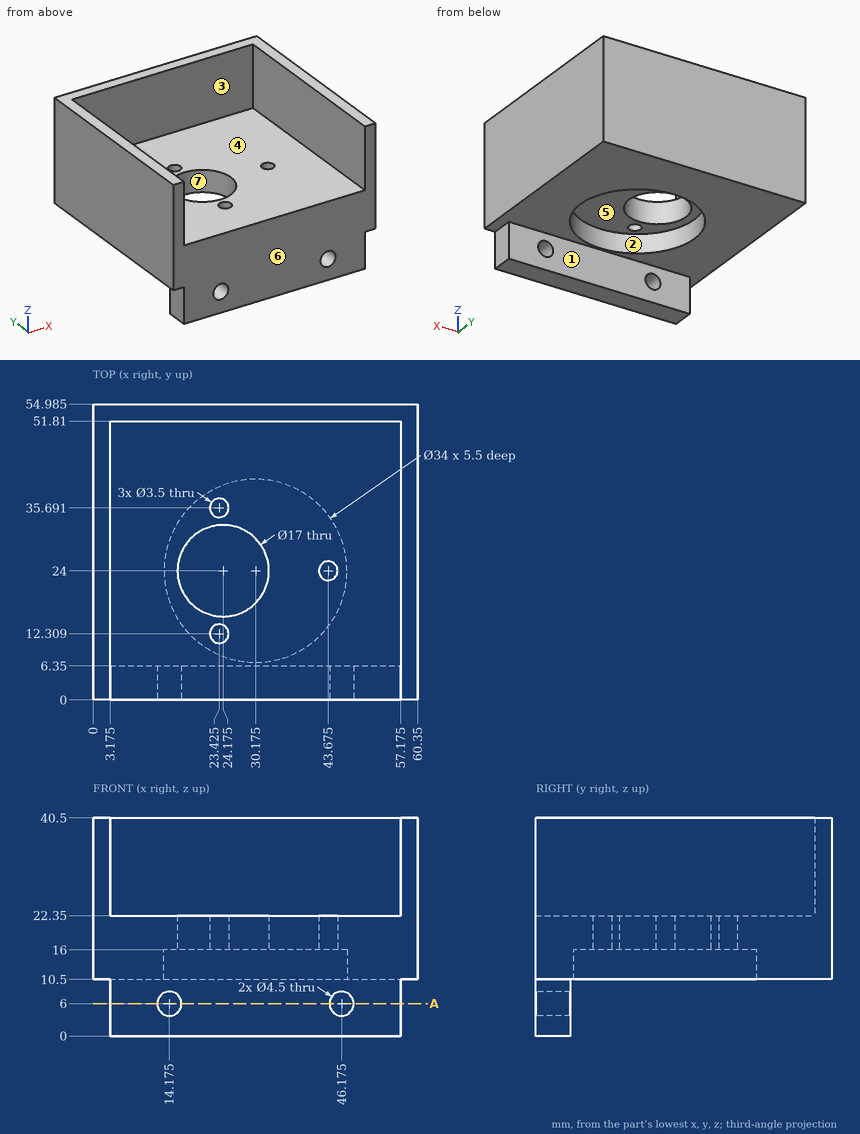
Geometry check sheet. Reference: drawing and pictorial views, mm from the part's lowest x, y, z. A direction names the side the tool comes from. Coordinates: 2 decimals unless noted, no trailing zeros. Write item = value, one per line. Start each with the question number.
1. Mould release check, pull along Y, two halves, no side actions. Record for the marked faces 4, 5, 6 and 7: pulls with the +Y half, pulls with the -Y half, needs draft (parallel to the pull), parting line crosses it, or undercut.
2. Sectioned sample at A-A (z = 6). State how many separate pieces and enclosed holes the cut face has, then the cut area to 3 significant figures.
3. Thickness scan on probe 1 along X at (y, z) = (3.5, 6) (1 decimal); probe 2 along Z at (x, y) = (10, 10.5); probe 3 along Z at (x, y) = (45, 21). Record the ranges inside material, lowest first.
4. Go/stop test with flat-tipped pins: pin 1 (2 mm diameter, centred on x = 23.42, y = 35.69, fed in from -Z); pin 2 (3 mm diameter, centred on x = 29, z = 5, fed in from +Y); pin 3 (5.5 mm diameter, centred on x = 23.42, y = 12.31, fed in from +Z); pin 4 (10 mm diameter, centred on x = 27.5, y = 28.5, fed in from -Z). Record where each tip stops, or that it passes through.
5. Tool access check on the marked faces 1, 2 and 3. Record the directions out of +Z, -Z, +X, -X, +Y, -Y that give a thin tool (end or side, any length) a straight path to the whole face; none if there is none.
The answers:
q1.face_4 = needs draft
q1.face_5 = undercut
q1.face_6 = pulls with the -Y half
q1.face_7 = undercut
q2.separate_pieces = 3
q2.enclosed_holes = 0
q2.area = 286 mm²
q3.probe_1 = 3.2 to 11.9, 16.4 to 43.9, 48.4 to 57.2
q3.probe_2 = 10.5 to 22.35
q3.probe_3 = 16 to 22.35
q4.pin_1 = through
q4.pin_2 = 6.35
q4.pin_3 = 22.35
q4.pin_4 = 16
q5.face_1 = -Z, +X, -X, +Y
q5.face_2 = -Z
q5.face_3 = +Z, -Y
